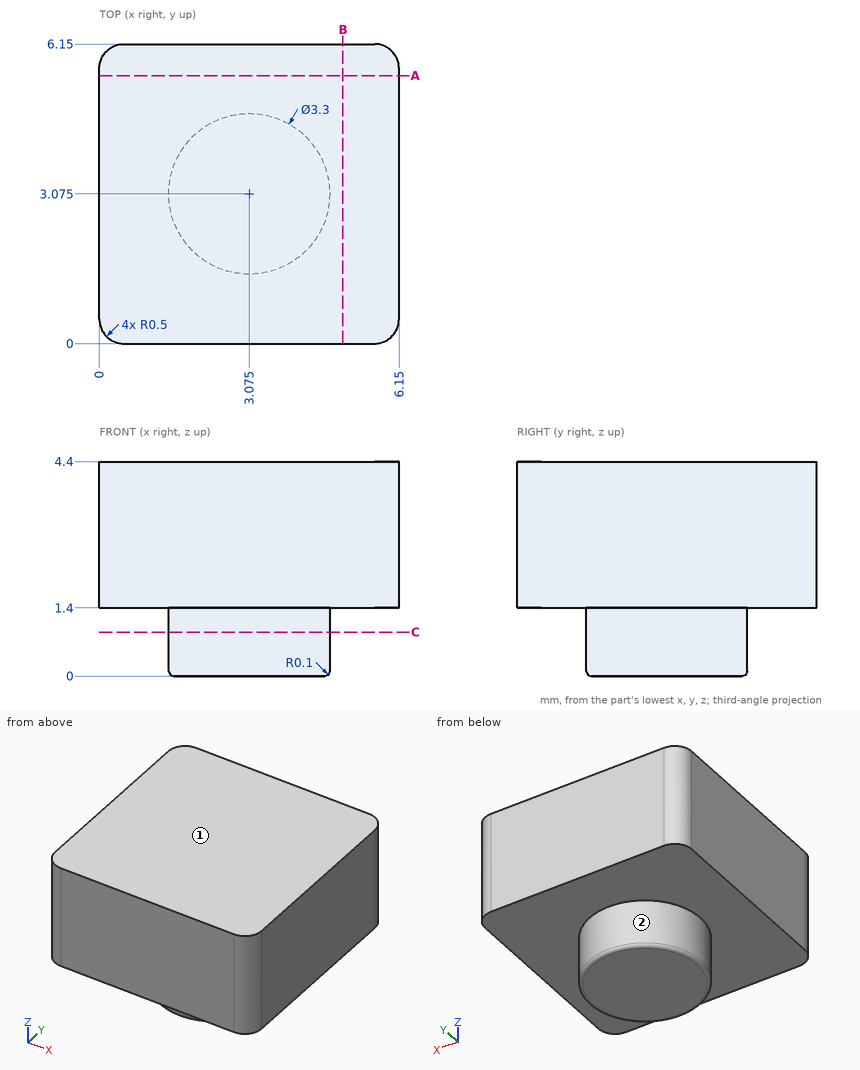
Verification items for this drawing (mm, ordinates from the low corner). A direction names the side the tool comes from. Coordinates: 2 decimals unless noted, no trailing zeros. Order: outer loops, then holes, each group sorted by start corner. A loop starts at its lowest first (then second) coordinate and runs counter-clockwise, first axis right, second up.
Q1. Tool access check on the marked faces 1 and 2. Record the directions out of +Z, -Z, +X, -X, +Y, -Y that give a thin tool (end or side, any length) a straight path to the whole face; none if there is none.
Reply:
face 1: +Z, +X, -X, +Y, -Y
face 2: -Z
Q2. Sectioned sample at C-C on z = 0.9. Record the cut outline in (x, y) (3 decimals).
Reply:
outline: circle Ø3.3 at (3.075, 3.075)
Q3. Thickness scan on probe 1 along Z at (x, y) = (3, 0.75); probe 2 along Y at (x, z) = (5.75, 4.15); probe 3 along Y at (x, z) = (1.75, 0.95). Record the ranges inside material, lowest first.
Reply:
probe 1: z = 1.4 to 4.4
probe 2: y = 0.01 to 6.14
probe 3: y = 2.09 to 4.06
Q4. Sectioned sample at A-A on y = 5.5. Record the cut outline in (x, z), and give its area (4 significant figures).
Reply:
outline: (0, 1.4) - (6.15, 1.4) - (6.15, 4.4) - (0, 4.4) - close
area: 18.45 mm2
